Verification items for this drawing (mm, ordinates from the low corner). Round coordinates to 2 decimals unless told otherwise and drop trailing zeros. Order: outer loops, then holes, each group sorted by start corner. A loop starts at its lowest first (then second) coordinate and runs counter-clockwise, first axis right, second up. Notation, with made-up numbers: (1.25, 29) -> (37.25, 29) arc R22 ccw to (37.25, 40) -> close; hole circle Ø4 at (86, 39.5). An arc over 180 degrees is marked (long way). Use a Markdown table: item, result. Add a question column.
Item 1: Sectioned sample at A-A, the plane y = 0.7. Record the cut outline in (x, z).
Item 2: Sectioned sample at D-D, the plane z = 46. Record the cut outline in (x, y) (1 decimal).
Item 3: Sectioned sample at B-B, the plane x = 32.5. Record the cut outline in (y, z).
Item 4: Sectioned sample at C-C, the plane z = 7.5. Record the cut outline in (x, y) (1 decimal).
Item 5: Material ranges on probe 1 along X at (y, z) = (1.2, 29); probe 2 along X at (y, z) = (1, 27.5); probe 3 along X at (y, z) = (0.95, 49), recorded low to high. Write a range as [from, to].
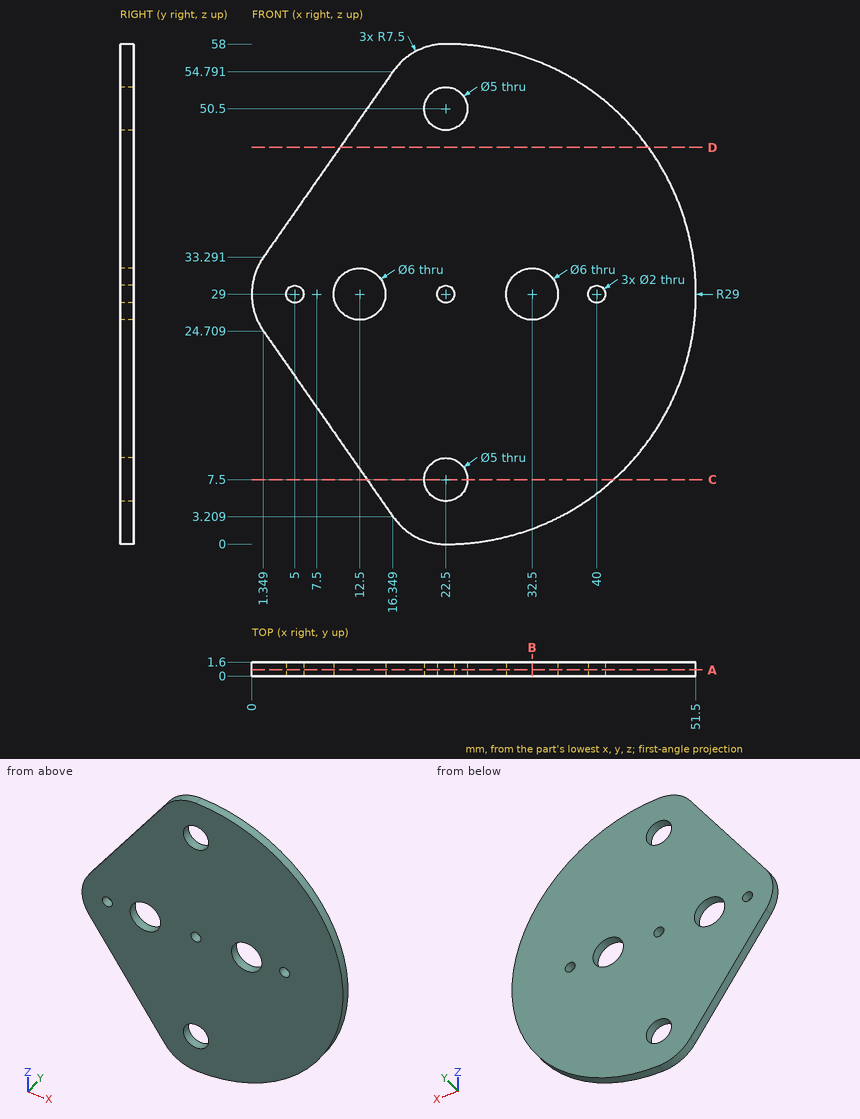
Found:
| question | item | result |
|---|---|---|
| 1 | outline | (1.35, 24.71) -> (16.35, 3.21) arc R7.5 ccw to (22.5, 0) arc R29 ccw to (22.5, 58) arc R7.5 ccw to (16.35, 54.79) -> (1.35, 33.29) arc R7.5 ccw to start; hole circle Ø2 at (5, 29); hole circle Ø6 at (12.5, 29); hole circle Ø5 at (22.5, 7.5); hole circle Ø5 at (22.5, 50.5); hole circle Ø2 at (22.5, 29); hole circle Ø6 at (32.5, 29); hole circle Ø2 at (40, 29) |
| 2 | outline | (10.2, 0) -> (46, 0) -> (46, 1.6) -> (10.2, 1.6) -> close |
| 3 | outline | (0, 1.78) -> (1.6, 1.78) -> (1.6, 26) -> (0, 26) -> close; (0, 32) -> (1.6, 32) -> (1.6, 56.22) -> (0, 56.22) -> close |
| 4 | outline | (13.4, 0) -> (20, 0) -> (20, 1.6) -> (13.4, 1.6) -> close; (25, 0) -> (42, 0) -> (42, 1.6) -> (25, 1.6) -> close |
| 5 | probe 1 | x = [0, 4], [6, 9.5], [15.5, 21.5], [23.5, 29.5], [35.5, 39], [41, 51.5] |
| 5 | probe 2 | x = [0.15, 9.9], [15.1, 29.9], [35.1, 51.46] |
| 5 | probe 3 | x = [12.31, 20.5], [24.5, 43.5] |
